Can you work these out from the drawing? Everything is in mm from the part's minimum corner. A direction names the side the tool comes from. Round coordinates to 2 decimals unless told otherwise and drop trailing zeros. Write each loop counter-clockwise with the first axis right and the second up, starting at its lowest first coordinate (ties: lowest second). Pieces come first, ordered by that corner, then holes. Notation, with made-up numbers: (85.25, -4.5) - (119.25, -4.5) arc R28 ccw to (119.25, 13.5) - close; hole circle Ø6 at (-11, 54.25). An arc over 180 degrees is marked (long way). One line per item, written item: value. Start each with the question number.
Item 1: Imagine slicing it at C-C, the plane x = 12.25. Please give me the cut outline in (y, z).
Item 2: Imagine slicing it at B-B, the plane z = 3.75. Please give me the cut outline in (x, y).
Item 3: If I drill on line 1 (Z direction, x = 10, y = 4.9); line 2 (Z direction, x = 9, y = 5.4); line 3 (Z direction, x = 2, y = 3) (1 decimal), over which ranges is the centre line in solid material (lowest first)?
Item 4: Imagine slicing it at A-A, the plane y = 5.1. Please give me the cut outline in (x, z), then the cut area to 3 significant figures.
Item 5: For the marked faces 1 and 2, which set-ups out of +Z, -Z, +X, -X, +Y, -Y let a thin tool reach every point of the face, with its end or its side?
Item 6: Imagine slicing it at D-D, the plane y = 4.1. Please give me the cut outline in (x, z).
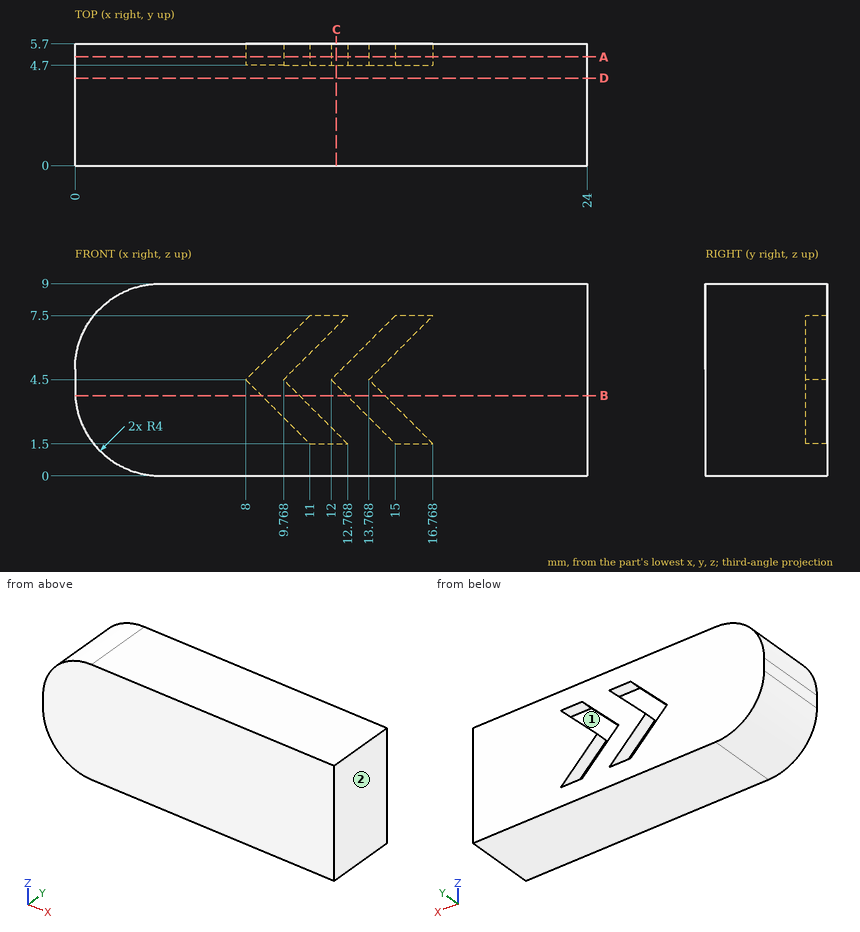
Values follow:
1. outline: (0, 0) - (5.7, 0) - (5.7, 1.5) - (4.7, 1.5) - (4.7, 2.02) - (5.7, 2.02) - (5.7, 4.25) - (4.7, 4.25) - (4.7, 4.75) - (5.7, 4.75) - (5.7, 6.98) - (4.7, 6.98) - (4.7, 7.5) - (5.7, 7.5) - (5.7, 9) - (0, 9) - close
2. outline: (0.01, 0) - (24, 0) - (24, 5.7) - (14.52, 5.7) - (14.52, 4.7) - (12.75, 4.7) - (12.75, 5.7) - (10.52, 5.7) - (10.52, 4.7) - (8.75, 4.7) - (8.75, 5.7) - (0.01, 5.7) - close
3. line 1: z = 0 to 2.5, 4.27 to 4.73, 6.5 to 9
3. line 2: z = 0 to 3.5, 5.5 to 9
3. line 3: z = 0.5 to 8.5
4. outline: (0, 4) arc R4 ccw to (4, 0) - (24, 0) - (24, 9) - (4, 9) arc R4 ccw to (0, 5) - close; hole (8, 4.5) - (11, 1.5) - (12.77, 1.5) - (9.77, 4.5) - (12.77, 7.5) - (11, 7.5) - close; hole (12, 4.5) - (15, 1.5) - (16.77, 1.5) - (13.77, 4.5) - (16.77, 7.5) - (15, 7.5) - close
4. area: 188 mm^2
5. face 1: +Y
5. face 2: +Z, -Z, +X, +Y, -Y
6. outline: (0, 4) arc R4 ccw to (4, 0) - (24, 0) - (24, 9) - (4, 9) arc R4 ccw to (0, 5) - close
